Autodesk Fusion 360 part; units mm, degrees
sketch "Esboço1" plane through (0, 0, 0) normal (0, 0, 1) x (1, 0, 0)
  line L0 (9.5, 9.5) -> (-9.5, 9.5)
  line L1 (-9.5, 9.5) -> (-9.5, -9.5)
  line L2 (-9.5, -9.5) -> (9.5, -9.5)
  line L3 (9.5, -9.5) -> (9.5, 9.5)
  line L4 (9.5, 9.5) -> (-9.5, -9.5) construction
  line L5 (-9.5, 9.5) -> (9.5, -9.5) construction
  circle A0 centre (0, 0) radius 6.5
  line L6 (-9.5, 9.5) -> (-7.5, 9.5)
  line L7 (-7.5, 9.5) -> (-7.5, 7.5)
  line L8 (-7.5, 7.5) -> (-9.5, 7.5)
  line L9 (-9.5, 7.5) -> (-9.5, 9.5)
  line L10 (9.5, 9.5) -> (7.5, 9.5)
  line L11 (7.5, 9.5) -> (7.5, 7.5)
  line L12 (7.5, 7.5) -> (9.5, 7.5)
  line L13 (9.5, 7.5) -> (9.5, 9.5)
  line L14 (-9.5, -9.5) -> (-7.5, -9.5)
  line L15 (-7.5, -9.5) -> (-7.5, -7.5)
  line L16 (-7.5, -7.5) -> (-9.5, -7.5)
  line L17 (-9.5, -7.5) -> (-9.5, -9.5)
  line L18 (9.5, -9.5) -> (7.5, -9.5)
  line L19 (7.5, -9.5) -> (7.5, -7.5)
  line L20 (7.5, -7.5) -> (9.5, -7.5)
  line L21 (9.5, -7.5) -> (9.5, -9.5)
  line L22 (-9.5, 9.5) -> (-7.5, 9.5)
  line L23 (-7.5, 9.5) -> (-7.5, 49.5)
  line L24 (-7.5, 49.5) -> (-9.5, 49.5)
  line L25 (-9.5, 49.5) -> (-9.5, 9.5)
  line L26 (9.5, 9.5) -> (7.5, 9.5)
  line L27 (7.5, 9.5) -> (7.5, 49.5)
  line L28 (7.5, 49.5) -> (9.5, 49.5)
  line L29 (9.5, 49.5) -> (9.5, 9.5)
  line L30 (-9.5, 49.5) -> (9.5, 49.5)
  line L31 (9.5, 49.5) -> (9.5, 61.5)
  line L32 (9.5, 61.5) -> (-9.5, 61.5)
  line L33 (-9.5, 61.5) -> (-9.5, 49.5)
  line L34 (-9.5, 61.5) -> (9.5, 49.5) construction
  circle A1 centre (0, 55.5) radius 2.5
  line L35 (-7.5, 9.5) -> (7.5, 9.5)
  line L36 (7.5, 9.5) -> (7.5, 15.5)
  line L37 (7.5, 15.5) -> (-7.5, 15.5)
  line L38 (-7.5, 15.5) -> (-7.5, 9.5)
  line L39 (-7.5, 15.5) -> (7.5, 15.5)
  line L40 (7.5, 15.5) -> (7.5, 17.5)
  line L41 (7.5, 17.5) -> (-7.5, 17.5)
  line L42 (-7.5, 17.5) -> (-7.5, 15.5)
  line L43 (-7.5, 17.5) -> (7.5, 17.5)
  line L44 (7.5, 17.5) -> (7.5, 25.5)
  line L45 (7.5, 25.5) -> (-7.5, 25.5)
  line L46 (-7.5, 25.5) -> (-7.5, 17.5)
  line L47 (-7.5, 25.5) -> (7.5, 25.5)
  line L48 (7.5, 25.5) -> (7.5, 27.5)
  line L49 (7.5, 27.5) -> (-7.5, 27.5)
  line L50 (-7.5, 27.5) -> (-7.5, 25.5)
  line L51 (-7.5, 27.5) -> (7.5, 27.5)
  line L52 (7.5, 27.5) -> (7.5, 35.5)
  line L53 (7.5, 35.5) -> (-7.5, 35.5)
  line L54 (-7.5, 35.5) -> (-7.5, 27.5)
  line L55 (-7.5, 35.5) -> (7.5, 35.5)
  line L56 (7.5, 35.5) -> (7.5, 37.5)
  line L57 (7.5, 37.5) -> (-7.5, 37.5)
  line L58 (-7.5, 37.5) -> (-7.5, 35.5)
  line L59 (9.5, 9.5) -> (49.5, 9.5)
  line L60 (49.5, 9.5) -> (49.5, 7.5)
  line L61 (49.5, 7.5) -> (9.5, 7.5)
  line L62 (9.5, 7.5) -> (9.5, 9.5)
  line L63 (9.5, -9.5) -> (49.5, -9.5)
  line L64 (49.5, -9.5) -> (49.5, -7.5)
  line L65 (49.5, -7.5) -> (9.5, -7.5)
  line L66 (9.5, -7.5) -> (9.5, -9.5)
  line L67 (49.5, 9.5) -> (61.5, 9.5)
  line L68 (61.5, 9.5) -> (61.5, -9.5)
  line L69 (61.5, -9.5) -> (49.5, -9.5)
  line L70 (49.5, -9.5) -> (49.5, 9.5)
  line L71 (49.5, 9.5) -> (61.5, -9.5) construction
  circle A2 centre (55.5, 0) radius 2.5
  line L72 (9.5, 7.5) -> (15.5, 7.5)
  line L73 (15.5, 7.5) -> (15.5, -7.5)
  line L74 (15.5, -7.5) -> (9.5, -7.5)
  line L75 (9.5, -7.5) -> (9.5, 7.5)
  line L76 (15.5, 7.5) -> (17.5, 7.5)
  line L77 (17.5, 7.5) -> (17.5, -7.5)
  line L78 (17.5, -7.5) -> (15.5, -7.5)
  line L79 (15.5, -7.5) -> (15.5, 7.5)
  line L80 (17.5, 7.5) -> (25.5, 7.5)
  line L81 (25.5, 7.5) -> (25.5, -7.5)
  line L82 (25.5, -7.5) -> (17.5, -7.5)
  line L83 (17.5, -7.5) -> (17.5, 7.5)
  line L84 (25.5, 7.5) -> (27.5, 7.5)
  line L85 (27.5, 7.5) -> (27.5, -7.5)
  line L86 (27.5, -7.5) -> (25.5, -7.5)
  line L87 (25.5, -7.5) -> (25.5, 7.5)
  line L88 (27.5, 7.5) -> (35.5, 7.5)
  line L89 (35.5, 7.5) -> (35.5, -7.5)
  line L90 (35.5, -7.5) -> (27.5, -7.5)
  line L91 (27.5, -7.5) -> (27.5, 7.5)
  line L92 (35.5, 7.5) -> (37.5, 7.5)
  line L93 (37.5, 7.5) -> (37.5, -7.5)
  line L94 (37.5, -7.5) -> (35.5, -7.5)
  line L95 (35.5, -7.5) -> (35.5, 7.5)
  line L96 (-9.5, -9.5) -> (-7.5, -9.5)
  line L97 (-7.5, -9.5) -> (-7.5, -49.5)
  line L98 (-7.5, -49.5) -> (-9.5, -49.5)
  line L99 (-9.5, -49.5) -> (-9.5, -9.5)
  line L100 (9.5, -9.5) -> (7.5, -9.5)
  line L101 (7.5, -9.5) -> (7.5, -49.5)
  line L102 (7.5, -49.5) -> (9.5, -49.5)
  line L103 (9.5, -49.5) -> (9.5, -9.5)
  line L104 (-9.5, -49.5) -> (9.5, -49.5)
  line L105 (9.5, -49.5) -> (9.5, -61.5)
  line L106 (9.5, -61.5) -> (-9.5, -61.5)
  line L107 (-9.5, -61.5) -> (-9.5, -49.5)
  line L108 (-9.5, -49.5) -> (9.5, -61.5) construction
  circle A3 centre (0, -55.5) radius 2.5
  line L109 (-9.5, -9.5) -> (9.5, -9.5)
  line L110 (9.5, -9.5) -> (9.5, -15.5)
  line L111 (9.5, -15.5) -> (-9.5, -15.5)
  line L112 (-9.5, -15.5) -> (-9.5, -9.5)
  line L113 (-9.5, -15.5) -> (9.5, -15.5)
  line L114 (9.5, -15.5) -> (9.5, -17.5)
  line L115 (9.5, -17.5) -> (-9.5, -17.5)
  line L116 (-9.5, -17.5) -> (-9.5, -15.5)
  line L117 (-9.5, -17.5) -> (9.5, -17.5)
  line L118 (9.5, -17.5) -> (9.5, -25.5)
  line L119 (9.5, -25.5) -> (-9.5, -25.5)
  line L120 (-9.5, -25.5) -> (-9.5, -17.5)
  line L121 (-9.5, -25.5) -> (9.5, -25.5)
  line L122 (9.5, -25.5) -> (9.5, -27.5)
  line L123 (9.5, -27.5) -> (-9.5, -27.5)
  line L124 (-9.5, -27.5) -> (-9.5, -25.5)
  line L125 (-9.5, -27.5) -> (9.5, -27.5)
  line L126 (9.5, -27.5) -> (9.5, -35.5)
  line L127 (9.5, -35.5) -> (-9.5, -35.5)
  line L128 (-9.5, -35.5) -> (-9.5, -27.5)
  line L129 (-9.5, -35.5) -> (9.5, -35.5)
  line L130 (9.5, -35.5) -> (9.5, -37.5)
  line L131 (9.5, -37.5) -> (-9.5, -37.5)
  line L132 (-9.5, -37.5) -> (-9.5, -35.5)
  line L133 (-9.5, 9.5) -> (-49.5, 9.5)
  line L134 (-49.5, 9.5) -> (-49.5, 7.5)
  line L135 (-49.5, 7.5) -> (-9.5, 7.5)
  line L136 (-9.5, 7.5) -> (-9.5, 9.5)
  line L137 (-9.5, -9.5) -> (-49.5, -9.5)
  line L138 (-49.5, -9.5) -> (-49.5, -7.5)
  line L139 (-49.5, -7.5) -> (-9.5, -7.5)
  line L140 (-9.5, -7.5) -> (-9.5, -9.5)
  line L141 (-49.5, -9.5) -> (-61.5, -9.5)
  line L142 (-61.5, -9.5) -> (-61.5, 9.5)
  line L143 (-61.5, 9.5) -> (-49.5, 9.5)
  line L144 (-49.5, 9.5) -> (-49.5, -9.5)
  line L145 (-61.5, 9.5) -> (-49.5, -9.5) construction
  circle A4 centre (-55.5, 0) radius 2.5
  line L146 (-9.5, 9.5) -> (-15.5, 9.5)
  line L147 (-15.5, 9.5) -> (-15.5, -9.5)
  line L148 (-15.5, -9.5) -> (-9.5, -9.5)
  line L149 (-9.5, -9.5) -> (-9.5, 9.5)
  line L150 (-15.5, 9.5) -> (-17.5, 9.5)
  line L151 (-17.5, 9.5) -> (-17.5, -9.5)
  line L152 (-17.5, -9.5) -> (-15.5, -9.5)
  line L153 (-15.5, -9.5) -> (-15.5, 9.5)
  line L154 (-17.5, 9.5) -> (-25.5, 9.5)
  line L155 (-25.5, 9.5) -> (-25.5, -9.5)
  line L156 (-25.5, -9.5) -> (-17.5, -9.5)
  line L157 (-17.5, -9.5) -> (-17.5, 9.5)
  line L158 (-25.5, 9.5) -> (-27.5, 9.5)
  line L159 (-27.5, 9.5) -> (-27.5, -9.5)
  line L160 (-27.5, -9.5) -> (-25.5, -9.5)
  line L161 (-25.5, -9.5) -> (-25.5, 9.5)
  line L162 (-27.5, 9.5) -> (-35.5, 9.5)
  line L163 (-35.5, 9.5) -> (-35.5, -9.5)
  line L164 (-35.5, -9.5) -> (-27.5, -9.5)
  line L165 (-27.5, -9.5) -> (-27.5, 9.5)
  line L166 (-35.5, 9.5) -> (-37.5, 9.5)
  line L167 (-37.5, 9.5) -> (-37.5, -9.5)
  line L168 (-37.5, -9.5) -> (-35.5, -9.5)
  line L169 (-35.5, -9.5) -> (-35.5, 9.5)
  dimension "d1" = 19
  dimension "d2" = 19
  dimension "d3" = 13
  dimension "d4" = 2
  dimension "d5" = 2
  dimension "d6" = 2
  dimension "d7" = 2
  dimension "d8" = 2
  dimension "d9" = 2
  dimension "d10" = 2
  dimension "d11" = 2
  dimension "d13" = 2
  dimension "d14" = 40
  dimension "d15" = 2
  dimension "d16" = 40
  dimension "d17" = 19
  dimension "d18" = 12
  dimension "d19" = 5
  dimension "d20" = 15
  dimension "d21" = 6
  dimension "d22" = 2
  dimension "d23" = 8
  dimension "d24" = 2
  dimension "d25" = 8
  dimension "d26" = 2
  dimension "d27" = 40
  dimension "d28" = 2
  dimension "d29" = 40
  dimension "d30" = 2
  dimension "d31" = 12
  dimension "d32" = 19
  dimension "d33" = 5
  dimension "d34" = 6
  dimension "d35" = 2
  dimension "d36" = 8
  dimension "d37" = 15
  dimension "d38" = 2
  dimension "d39" = 8
  dimension "d40" = 2
  dimension "d41" = 40
  dimension "d42" = 2
  dimension "d43" = 40
  dimension "d44" = 12
  dimension "d45" = 5
  dimension "d46" = 6
  dimension "d47" = 2
  dimension "d48" = 8
  dimension "d49" = 2
  dimension "d50" = 8
  dimension "d51" = 2
  dimension "d52" = 40
  dimension "d53" = 2
  dimension "d54" = 40
  dimension "d55" = 2
  dimension "d56" = 12
  dimension "d57" = 19
  dimension "d58" = 5
  dimension "d59" = 6
  dimension "d60" = 2
  dimension "d61" = 8
  dimension "d62" = 2
  dimension "d63" = 8
  dimension "d64" = 2
extrude "Extrusão1" add sketch "Esboço1" along normal blind 8 contours L0 L3 L10 L11 L12 L13 L26 L62 | L3 L13 L59 L60 L61 L62 L70 L72 L76 L80 L84 L88 L92 | L0 L10 L26 L27 L28 L29 L30 L36 L40 L44 L48 L52 L56 | L0 L1 L2 L3 L7 L8 L11 L12 L15 L16 L19 L20 L35 L75 L109 L149 | L24 L28 L30 L31 L32 L33 | L60 L64 L67 L68 L69 L70 | L0 L1 L6 L7 L8 L9 L22 L136 L149 | L0 L6 L22 L23 L24 L25 L30 L38 L42 L46 L50 L54 L58 | L23 L27 L37 L39 L40 L41 L42 L43 | L3 L21 L63 L64 L65 L66 L70 L74 L78 L82 L86 L90 L94 | L2 L3 L18 L19 L20 L21 L66 L100 L109 | L61 L65 L73 L76 L77 L78 L79 L83 | L1 L9 L133 L135 L136 L146 L147 L149 L153 | L2 L18 L100 L101 L103 L109 L110 L111 L113 | L23 L27 L53 L55 L56 L57 L58 | L61 L65 L89 L92 L93 L94 L95 | L133 L135 L147 L150 L151 L153 L157 | L23 L27 L45 L47 L48 L49 L50 L51 | L101 L103 L111 L113 L114 L115 L117 | L61 L65 L81 L84 L85 L86 L87 L91 | L1 L2 L14 L15 L16 L17 L96 L109 L140 L149 | L1 L17 L137 L139 L140 L147 L148 L149 L153 | L135 L139 L147 L151 L153 L157 | L133 L135 L151 L154 L155 L157 L161 | L2 L14 L96 L97 L99 L109 L111 L112 L113 | L97 L101 L111 L113 L115 L117 | L101 L103 L115 L117 L118 L119 L121 | L137 L139 L147 L151 L152 L153 L157 | L133 L135 L155 L158 L159 L161 L165 | L97 L99 L111 L113 L115 L116 L117 | L101 L103 L119 L121 L122 L123 L125 | L137 L139 L151 L155 L156 L157 L161 | L135 L139 L155 L159 L161 L165 | L133 L135 L159 L162 L163 L165 L169 | L97 L99 L115 L117 L119 L120 L121 | L97 L101 L119 L121 L123 L125 | L101 L103 L123 L125 L126 L127 L129 | L137 L139 L155 L159 L160 L161 L165 | L133 L135 L163 L166 L167 L169 | L97 L99 L119 L121 L123 L124 L125 | L101 L103 L127 L129 L130 L131 | L137 L139 L159 L163 L164 L165 L169 | L135 L139 L163 L167 L169 | L133 L134 L135 L144 L167 | L97 L99 L123 L125 L127 L128 L129 | L97 L101 L127 L129 L131 | L101 L102 L103 L104 L131 | L137 L139 L163 L167 L168 L169 | L134 L138 L141 L142 L143 L144 | L97 L99 L127 L129 L131 L132 | L98 L102 L104 L105 L106 L107 | L137 L138 L139 L144 L167 | L97 L98 L99 L104 L131
extrude "Extrusão2" add sketch "Esboço1" against normal blind 4 contours L0 L3 L10 L11 L12 L13 L26 L62 | L3 L13 L59 L60 L61 L62 L70 L72 L76 L80 L84 L88 L92 | L0 L10 L26 L27 L28 L29 L30 L36 L40 L44 L48 L52 L56 | L24 L28 L30 L31 L32 L33 | L60 L64 L67 L68 L69 L70 | L0 L1 L6 L7 L8 L9 L22 L136 L149 | L0 L6 L22 L23 L24 L25 L30 L38 L42 L46 L50 L54 L58 | L3 L21 L63 L64 L65 L66 L70 L74 L78 L82 L86 L90 L94 | L2 L3 L18 L19 L20 L21 L66 L100 L109 | L1 L9 L133 L135 L136 L146 L147 L149 L153 | L2 L18 L100 L101 L103 L109 L110 L111 L113 | L133 L135 L147 L150 L151 L153 L157 | L101 L103 L111 L113 L114 L115 L117 | L1 L2 L14 L15 L16 L17 L96 L109 L140 L149 | L1 L17 L137 L139 L140 L147 L148 L149 L153 | L133 L135 L151 L154 L155 L157 L161 | L2 L14 L96 L97 L99 L109 L111 L112 L113 | L101 L103 L115 L117 L118 L119 L121 | L137 L139 L147 L151 L152 L153 L157 | L133 L135 L155 L158 L159 L161 L165 | L97 L99 L111 L113 L115 L116 L117 | L101 L103 L119 L121 L122 L123 L125 | L137 L139 L151 L155 L156 L157 L161 | L133 L135 L159 L162 L163 L165 L169 | L97 L99 L115 L117 L119 L120 L121 | L101 L103 L123 L125 L126 L127 L129 | L137 L139 L155 L159 L160 L161 L165 | L133 L135 L163 L166 L167 L169 | L97 L99 L119 L121 L123 L124 L125 | L101 L103 L127 L129 L130 L131 | L137 L139 L159 L163 L164 L165 L169 | L133 L134 L135 L144 L167 | L97 L99 L123 L125 L127 L128 L129 | L101 L102 L103 L104 L131 | L137 L139 L163 L167 L168 L169 | L134 L138 L141 L142 L143 L144 | L97 L99 L127 L129 L131 L132 | L98 L102 L104 L105 L106 L107 | L137 L138 L139 L144 L167 | L97 L98 L99 L104 L131
Can you work these out from the model? Positions are in its coordinate system, mm. A direction names the side the tool comes from. Round coordinates to 2 decimals unless told otherwise and drop trailing zeros. Loops run counter-clockwise (first coordinate to the right, second up) from the corner with the lowest first, then second, coordinate; pieces in that order, holes last. Notation, with made-up numbers: (79, 36) - (98, 36) arc R25 ccw to (98, 62) - close; hole circle Ø5 at (63, -1). An arc over 180 degrees is marked (long way). Use CSV: the item, a comma, the result in double quotes. Start each with the question number.
1) If we section it at D-D on x = 0: Count the separate pieces of the cut face and the enclosed holes in it, plus the area to 3 significant figures.
2) If we section it at C-C on z = -1.5: Write out the boundary of the cut face in (x, y), plus the area to 3 significant figures.
3) If we section it at A-A on y = 41.5: Write out the boundary of the cut face in (x, z).
4) We'd pull the mould along Y, two halves only. Please class faces 1 (the flat face through (-29, 7.5, 2)), 2 (the flat face through (0, 27.5, 4)), 3 (the flat face through (-35, -9.5, 2)), 4 (the flat face through (9.5, 36, 2)): released by +Y, released by -Y, zero draft, split by the parting line, or undercut.
5) For pin 1 Ø6 at (y, z) = (-42.5, -2.5) entering from -X; pin 2 Ø3.5 at (x, z) = (30.5, 3) entering from +Y; pin 3 Ø2 at (y, z) = (24.5, -2) entering from +X, each with a flat end and sliding along its axis, tell me the tip position at first contact or that it passes through.
6) For faces 5 (the flat face through (-15.5, 0, 4)), 6 (the flat face through (-9.5, 36, 2)), 7 (the flat face through (-9.5, -36, 2)), which set-ups out of +Z, -Z, +X, -X, +Y, -Y let a thin tool reach every point of the face, with its end or its side?
7) Please list where these lines run through material, in increasing order: probe 1 along Y at (x, z) = (0, -1.5); probe 2 along X at (y, z) = (-3, -1.75); probe 3 along Y at (x, z) = (37, -2). Write a range as [from, to].
Geometry results:
1,separate pieces,"12"
1,enclosed holes,"0"
1,area,"312 mm2"
2,outline,"(-61.5, -9.5) - (-9.5, -9.5) - (-9.5, -61.5) - (9.5, -61.5) - (9.5, -9.5) - (61.5, -9.5) - (61.5, 9.5) - (9.5, 9.5) - (9.5, 61.5) - (-9.5, 61.5) - (-9.5, 9.5) - (-61.5, 9.5) - close; hole circle Ø5 at (-55.5, 0); hole (-49.5, -7.5) - (-7.5, -7.5) - (-7.5, -49.5) - (7.5, -49.5) - (7.5, -7.5) - (49.5, -7.5) - (49.5, 7.5) - (7.5, 7.5) - (7.5, 49.5) - (-7.5, 49.5) - (-7.5, 7.5) - (-49.5, 7.5) - close; hole circle Ø5 at (0, -55.5); hole circle Ø5 at (0, 55.5); hole circle Ø5 at (55.5, 0)"
2,area,"1,490 mm2"
3,outline,"(-9.5, -4) - (-7.5, -4) - (-7.5, 8) - (-9.5, 8) - close; (7.5, -4) - (9.5, -4) - (9.5, 8) - (7.5, 8) - close"
4,face 1,"undercut"
4,face 2,"undercut"
4,face 3,"released by -Y"
4,face 4,"zero draft"
5,pin 1,"stops at x = -9.5"
5,pin 2,"stops at y = 9.5"
5,pin 3,"stops at x = 9.5"
6,face 5,"+Z, -Z"
6,face 6,"+Z, -Z, -X, +Y"
6,face 7,"+Z, -Z, -X, -Y"
7,probe 1,"y = [-61.5, -58], [-53, -49.5], [49.5, 53], [58, 61.5]"
7,probe 2,"x = [-61.5, -49.5], [49.5, 61.5]"
7,probe 3,"y = [-9.5, -7.5], [7.5, 9.5]"
